The listing builds one solid part. Answer for the finished solid, in the listing's coordinates (mm). A direction names the side the tool comes from. Coordinates: 2 decimals unless noted, no trailing zeros. Loops run counter-clockwise (first coordinate to the right, second up) from the corner with the lowest first, then second, coordinate; pieces in that order, holes last. Notation, with made-up numbers: (35, 28.25) - (53, 28.25) arc R37 ccw to (53, 64.25) - close; hole circle Ø5 at (-29.75, 41.5). An arc over 180 degrees is marked (long way). Put each result on its own line as item: value.
```python
from build123d import *

# Parameters (mm, degrees)
SKETCH_1_R               = 30
EXTRUDE_1_DEPTH          = 8
SKETCH_2_R               = 16.5
CUT_EXTRUDE_1_DEPTH      = 8
EXTRUDE_START            = 15
SKETCH_3_R               = 19
SKETCH_3_R_2             = 16.5
EXTRUDE_2_DEPTH          = 15
CUT_EXTRUDE_2_DEPTH      = 26
CUT_EXTRUDE_2_DEPTH_BACK = 22
SKETCH_6_R               = 2


with BuildPart() as part:
    # 草图1 → 凸台-拉伸1 (new body)
    with BuildSketch(Plane(origin=(0, 0, 0), x_dir=(1, 0, 0), z_dir=(0, 1, 0))):
        with Locations(Location((0, 0, 0), (0, 0, 270))):
            Circle(SKETCH_1_R)
    extrude(amount=EXTRUDE_1_DEPTH)

    # 草图2 → 切除-拉伸1 (cut)
    with BuildSketch(Plane(origin=(0, 8, 0), x_dir=(1, 0, 0), z_dir=(0, 1, 0))):
        with Locations(Location((0, 0, 0), (0, 0, 270))):
            Circle(SKETCH_2_R)
    extrude(amount=-CUT_EXTRUDE_1_DEPTH, mode=Mode.SUBTRACT)

    # 草图3 → 凸台-拉伸2 (add)
    with BuildSketch(Plane(origin=(0, 8, 0), x_dir=(1, 0, 0), z_dir=(0, 1, 0)).offset(EXTRUDE_START)):
        with Locations(Location((0, 0, 0), (0, 0, 270))):
            Circle(SKETCH_3_R)
        with Locations(Location((0, 0, 0), (0, 0, 270))):
            Circle(SKETCH_3_R_2, mode=Mode.SUBTRACT)
    extrude(amount=-EXTRUDE_2_DEPTH)

    # 扫描1: sweep along a curve in space
    with BuildLine() as sweep_1_path:
        ThreePointArc((0, 8, 19), (13.435028843, 8, 13.435028843), (19, 8, 0))
        ThreePointArc((19, 8, 0), (13.435028843, 8, -13.435028843), (0, 8, -19))
        ThreePointArc((0, 8, -19), (-13.435028843, 8, -13.435028843), (-19, 8, 0))
        ThreePointArc((-19, 8, 0), (-13.435028843, 8, 13.435028843), (0, 8, 19))
    # 草图5 → 扫描1 (sweep)
    with BuildSketch(Plane.XY):
        Polygon((-19, 15.5), (-19, 8), (-26.5, 8), align=None)
    sweep(path=sweep_1_path.line)

    # 草图6 → 切除-拉伸2 (cut, two sides: drawn at the far end of the back side and taken through both)
    with BuildSketch(Plane.XY.offset(-CUT_EXTRUDE_2_DEPTH_BACK)):
        with Locations(Location((0, 19.65958907, 0), (0, 0, 180))):
            Circle(SKETCH_6_R)
    extrude(amount=CUT_EXTRUDE_2_DEPTH + CUT_EXTRUDE_2_DEPTH_BACK, mode=Mode.SUBTRACT)


solid = part.part
```
1) The part is cut by section C-C (y = 2.25). Give the vertices of the cut face in (x, z).
Found:
outline: circle Ø60 at (0, 0); hole circle Ø33 at (0, 0)
2) Each of these flat-tipped pins is pushed along its axis until it touches: pin 1 (18 mm diameter, centred on x = -9.5, z = -7, fed in from +Y); pin 2 (10 mm diameter, centred on y = 15, z = 8, fed in from -X); pin 3 (10 mm diameter, centred on x = 8.5, y = 19.5, fed in from -Z); pin 4 (3 mm diameter, centred on x = -23.5, z = -18, fed in from +Y). Where does it stop, or does it pass through?
Found:
pin 1: stops at y = 23
pin 2: stops at x = -23.39
pin 3: stops at z = -18.67
pin 4: stops at y = 8
3) Straight lines are drawn through the part: L1, parallel to Y at x = 19, z = -22.5; L2, parallel to X at y = 17.75, z = -0.5; L3, parallel to X at y = 4.75, z = 0. For each, find the intervals that lie inside material, in ascending order. Write a range as [from, to].
Found:
L1: y = [0, 8]
L2: x = [-18.99, -16.49], [16.49, 18.99]
L3: x = [-30, -16.5], [16.5, 30]
4) For a pull along Y with two mould halves and no side action, classify faces 3 (the face through (16, 23, -6)), 4 (the face through (1.32, 3.94, -29.97)), 5 (the face through (0.434, 21.612, -17.708)) as pulls with the +Y half, pulls with the -Y half, needs draft (parallel to the pull), parting line crosses it, or undercut.
Found:
face 3: pulls with the +Y half
face 4: needs draft
face 5: undercut
5) The part is cut by section A-A (y = 13). Give the vertices of the cut face in (x, z), and give its area (3 significant figures).
Found:
outline: circle Ø43 at (0, 0); hole circle Ø33 at (0, 0)
area: 597 mm^2
6) For faces 1 (the face through (5.71, 19.3, 18.12)), 2 (the face through (4.956, 11.661, 15.738)), determine the directions among +Z, -Z, +X, -X, +Y, -Y from which every point of the face is accessible in a straight line to the end or side of a thin tool.
Found:
face 1: +Y
face 2: +Y, -Y
7) The part is cut by section B-B (y = 20.5). Give the vertices of the cut face in (x, z), and give its area (3 significant figures).
Found:
outline: (-1.81, -18.91) - (-1.81, -16.4) arc R16.5 cw to (-1.81, 16.4) - (-1.81, 18.91) arc R19 ccw to start; (1.81, -18.91) arc R19 ccw to (1.81, 18.91) - (1.81, 16.4) arc R16.5 cw to (1.81, -16.4) - close
area: 261 mm^2
